For this review, take the finished solid that the model builds, in its own axes (mm). Coordinates: 2 decimals unless noted, no trailing zeros. Write each loop counter-clockwise with the first axis right and the second up, starting at its lowest first coordinate (ties: lowest second). Pieces come first, ordered by that corner, then holes. Notation, with made-up numbers: (33, 58) -> (80, 58) arc R15 ccw to (80, 80) -> close; hole circle Ø5 at (52.5, 26). An arc over 180 degrees is marked (long way). Put each result on its own line as item: value. Start each with the question number.
Item 1: To check wall thickness, follow L1, parallel to Y at x = 2.75, z = -3.5; L2, parallel to Z at x = 1.25, y = -4; L3, parallel to Y at x = 3, z = 0.5. State the ranges of each line that lie inside material, in increasing order.
Item 2: Consider section A-A on y = 0. Give the boundary of the cut face in (x, z), and give its area (3 significant figures).
Item 3: Insertion check: P1, Ø3, axis at x = -1, z = -8, coming from the +Y side; P2, Ø4, axis at x = -2.5, z = -31.5, coming from the -Y side; P3, Ø4, axis at x = 3.5, z = -3, coming from the +Y side; P4, Ø1, axis at x = -2, y = -19.5, coming from the -Z side. Each pin has a flat end and moves straight along its axis. Give the tip position at first contact, or say it passes through.
Item 4: The part is to be moulded in two halves that separate along Y. For faces 1 (the conical face through (-5.854, -23.246, 5.162)), 2 (the flat face through (0.057, -22.914, -29.062)), say which applies: +Y half, -Y half, draft (parallel to the pull), parting line (faces both ways), or undercut.
```python
from build123d import *

# Parameters (mm, degrees)
SKETCH1_R           = 40
SKETCH1_R_2         = 5
BOSS_EXTRUDE1_DEPTH = 6
CHAMFER2_SIZE       = 3
CHAMFER2_SIZE2      = 17.013845459
CHAMFER3_SIZE       = 3
CHAMFER3_SIZE2      = 17.013845459
CUT_EXTRUDE2_DEPTH  = 12
CIRPATTERN2_COUNT   = 33


with BuildPart() as part:
    # Sketch1 → Boss-Extrude1 (new body, symmetric)
    with BuildSketch(Plane(origin=(0, 0, 0), x_dir=(0, 0, -1), z_dir=(1, 0, 0))):
        Circle(SKETCH1_R)
        Circle(SKETCH1_R_2, mode=Mode.SUBTRACT)
    extrude(amount=BOSS_EXTRUDE1_DEPTH, both=True)

    # Chamfer2
    chamfer2_edges = [part.edges().sort_by_distance(p)[0] for p in [
        (6, 0, 40),
    ]]
    chamfer2_side = [part.faces().sort_by_distance(p)[0] for p in [
        (0, 0, 40),
    ]]
    chamfer(chamfer2_edges, length=CHAMFER2_SIZE, length2=CHAMFER2_SIZE2, reference=chamfer2_side[0])

    # Chamfer3
    chamfer3_edges = [part.edges().sort_by_distance(p)[0] for p in [
        (-6, 0, 40),
    ]]
    chamfer3_side = [part.faces().sort_by_distance(p)[0] for p in [
        (-1.5, 0, 40),
    ]]
    chamfer(chamfer3_edges, length=CHAMFER3_SIZE, length2=CHAMFER3_SIZE2, reference=chamfer3_side[0])

    # Sketch2 → Cut-Extrude2 (cut)
    with BuildSketch(Plane(origin=(6, 0, 0), x_dir=(0, 0, -1), z_dir=(1, 0, 0))):
        with BuildLine():
            Line((0, 34), (3.381435126, 39.856817441))
            ThreePointArc((3.381435126, 39.856817441), (0, 40.762870252), (-3.381435126, 39.856817441))
            Line((-3.381435126, 39.856817441), (0, 34))
        make_face()
    cut_extrude2 = extrude(amount=-CUT_EXTRUDE2_DEPTH, mode=Mode.SUBTRACT)

    # CirPattern2: Cut-Extrude2 ×33 about axis
    cirpattern2_axis = Axis((0, 0, 0), (1, 0, 0))
    for i in range(1, CIRPATTERN2_COUNT):
        add(cut_extrude2.rotate(cirpattern2_axis, i * 360 / CIRPATTERN2_COUNT), mode=Mode.SUBTRACT)


solid = part.part
```
Return value:
1. L1: -34.22 to -3.57, 3.57 to 39.85
1. L2: -35.75 to -3, 3 to 35.75
1. L3: -39.83 to -4.97, 4.97 to 34.87
2. outline: (-6, -22.99) -> (-3.51, -37.1) -> (3.51, -37.1) -> (6, -22.99) -> (6, -5) -> (-6, -5) -> close; (-6, 5) -> (6, 5) -> (6, 22.99) -> (3.51, 37.1) -> (-3.51, 37.1) -> (-6, 22.99) -> close
2. area: 700 mm^2
3. P1: y = 36.92
3. P2: y = -23.55
3. P3: y = 39.86
3. P4: z = -31.18
4. face 1: parting line
4. face 2: undercut
